```python
from build123d import *

# Parameters (mm, degrees)
BOSS_EXTRUDE1_DEPTH = 4
SKETCH4_W           = 21.88
SKETCH4_H           = 53
CUT_EXTRUDE1_DEPTH  = 4


with BuildPart() as part:
    # Layer1 → Boss-Extrude1 (new body)
    with BuildSketch(Plane(origin=(0, 0, 0), x_dir=(1, 0, 0), z_dir=(0, 1, 0))):
        with BuildLine():
            Line((27, 42), (11.25, 42))
            Line((11.25, 42), (-27, 42))
            ThreePointArc((-27, 42), (-37.606601718, 37.606601718), (-42, 27))
            Line((-42, 27), (-42, 21.5))
            Line((-42, 21.5), (-42, -21.5))
            Line((-42, -21.5), (-42, -27))
            ThreePointArc((-42, -27), (-37.606601718, -37.606601718), (-27, -42))
            Line((-27, -42), (11.25, -42))
            Line((11.25, -42), (27, -42))
            ThreePointArc((27, -42), (37.606601718, -37.606601718), (42, -27))
            Line((42, -27), (42, 27))
            ThreePointArc((42, 27), (37.606601718, 37.606601718), (27, 42))
        make_face()
    extrude(amount=BOSS_EXTRUDE1_DEPTH)

    # Sketch4 → Cut-Extrude1 (cut)
    with BuildSketch(Plane(origin=(0, 4, 0), x_dir=(1, 0, 0), z_dir=(0, 1, 0))):
        with Locations((31.06, 0)):
            Rectangle(SKETCH4_W, SKETCH4_H)
    extrude(amount=-CUT_EXTRUDE1_DEPTH, mode=Mode.SUBTRACT)


solid = part.part
```
Geometry: final body of the model. Coordinates: model frame, mm. A direction names the side the tool comes from. Coordinates: 2 decimals unless noted, no trailing zeros. Order: outer loops, then holes, each group sorted by start corner. A loop starts at its lowest first (then second) coordinate and runs counter-clockwise, first axis right, second up. Notation, with made-up numbers: (-11, 57) -> (22, 57) arc R12 ccw to (22, 72) -> close; hole circle Ø6 at (75.5, -18.75). An arc over 180 degrees is marked (long way). Write each question's results on one line, items separated by ' | '. Start each with the question number.
1) Set-up query: faces 1 (the flat face through (20.12, 2, 0)), 2 (the cylindrical face through (-37.72, 1.97, 37.49)). Return all of +Z, -Z, +X, -X, +Y, -Y with unobstructed straight access to the full face (end or side cutting, diameter ignored); none if empty.
2) First-contact query: pin 1 (2 mm diameter, centred on y = 3, z = -22, fed in from +X). Flat tip, straight axial feed; report the tip coordinate or a pass-through.
3) Cut plane B-B, the plane x = 34. Output: boundary loops of the cut face in (y, z).
4) Cut plane A-A, the plane y = 2.5. Output: boundary loops of the cut face in (x, z).
5) Material intervals for line 1 along Z through (x, y) = (25, 2.4); line 2 along X through (y, z) = (1.75, 7); line 3 along Z through (x, y) = (36, 3.5), sorted ascending.
6) Mould query, pull axis Z, two halves, no side actions, for faces 3 (the flat face through (0, 2, -42)), 4 (the flat face through (31, 2, 26.5)), 5 (the flat face through (-1, 0, -1)), 6 (the flat face through (31, 2, -26.5)). Classes: released by +Z, released by -Z, zero draft, split by the parting line, or undercut.
7) Cut plane C-C, the plane z = 23. Output: boundary loops of the cut face in (x, y).
8) Cut plane D-D, the plane x = -33. Output: boundary loops of the cut face in (y, z).
Checks:
1) face 1: +X, +Y, -Y | face 2: +Z, -X, +Y, -Y
2) pin 1: x = 20.12
3) outline: (0, -40.27) -> (4, -40.27) -> (4, -26.5) -> (0, -26.5) -> close; (0, 26.5) -> (4, 26.5) -> (4, 40.27) -> (0, 40.27) -> close
4) outline: (-42, -27) arc R15 ccw to (-27, -42) -> (27, -42) arc R15 ccw to (42, -27) -> (42, -26.5) -> (20.12, -26.5) -> (20.12, 26.5) -> (42, 26.5) -> (42, 27) arc R15 ccw to (27, 42) -> (-27, 42) arc R15 ccw to (-42, 27) -> close
5) line 1: -42 to -26.5, 26.5 to 42 | line 2: -42 to 20.12 | line 3: -39 to -26.5, 26.5 to 39
6) face 3: released by -Z | face 4: undercut | face 5: zero draft | face 6: undercut
7) outline: (-42, 0) -> (20.12, 0) -> (20.12, 4) -> (-42, 4) -> close
8) outline: (0, -40.75) -> (4, -40.75) -> (4, 40.75) -> (0, 40.75) -> close
